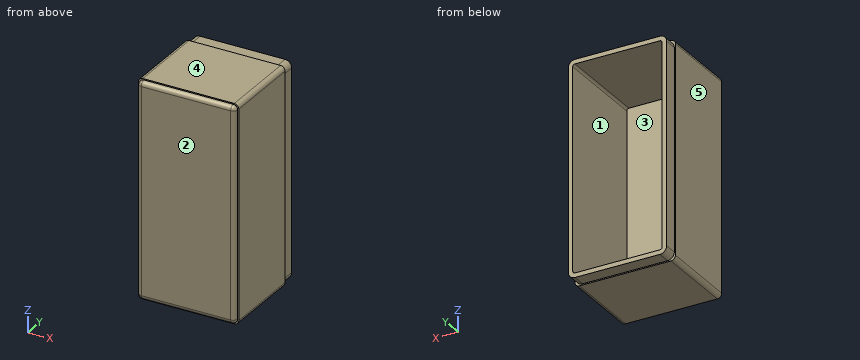
from build123d import *

# Parameters (mm, degrees)
SKETCH1_W           = 45
SKETCH1_H           = 97
BOSS_EXTRUDE1_DEPTH = 19
SKETCH2_W           = 44
SKETCH2_H           = 96
BOSS_EXTRUDE2_DEPTH = 6
SKETCH3_W           = 45
SKETCH3_H           = 97
SKETCH3_W_2         = 44
SKETCH3_H_2         = 96
CUT_EXTRUDE1_DEPTH  = 2
FILLET1_R           = 2
FILLET4_R           = 3
FILLET5_R           = 2
SHELL2_START        = -17
SHELL2_DEPTH        = 42
SHELL2_2_OUTLINE_W  = 41
SHELL2_2_OUTLINE_H  = 93
SHELL2_2_DEPTH      = 34
BOSS_EXTRUDE3_START = 34
SKETCH4_W           = 41
SKETCH4_H           = 93
BOSS_EXTRUDE3_DEPTH = 34


# Read off the part's stored shape, not the designer's step: Shell2
with BuildPart() as part:
    # Sketch1 → Boss-Extrude1 (new, symmetric)
    with BuildSketch(Plane(origin=(0, 0, 0), x_dir=(1, 0, 0), z_dir=(0, 1, 0))):
        Rectangle(SKETCH1_W, SKETCH1_H)
    extrude(amount=BOSS_EXTRUDE1_DEPTH, both=True)

    # Sketch2 → Boss-Extrude2 (add)
    with BuildSketch(Plane(origin=(0, 19, 0), x_dir=(1, 0, 0), z_dir=(0, 1, 0))):
        Rectangle(SKETCH2_W, SKETCH2_H)
    extrude(amount=BOSS_EXTRUDE2_DEPTH)

    # Sketch3 → Cut-Extrude1 (cut)
    with BuildSketch(Plane.XZ.offset(19)):
        Rectangle(SKETCH3_W, SKETCH3_H)
        Rectangle(SKETCH3_W_2, SKETCH3_H_2, mode=Mode.SUBTRACT)
    extrude(amount=-CUT_EXTRUDE1_DEPTH, mode=Mode.SUBTRACT)

    # Fillet1
    fillet1_edges = [part.edges().sort_by_distance(p)[0] for p in [
        (22, -19, 0),
        (22, -18, -48),
        (0, -19, -48),
        (-22, -18, -48),
        (-22, -19, 0),
        (-22, -18, 48),
        (0, -19, 48),
        (22, -18, 48),
    ]]
    fillet(fillet1_edges, radius=FILLET1_R - 0.0001)  # a hair under: the kernel refuses the full size

    # Fillet4
    fillet4_edges = [part.edges().sort_by_distance(p)[0] for p in [
        (22, 22, 48),
        (22, 22, -48),
        (-22, 22, -48),
        (-22, 22, 48),
    ]]
    fillet(fillet4_edges, radius=FILLET4_R)

    # Fillet5
    fillet5_edges = [part.edges().sort_by_distance(p)[0] for p in [
        (22.5, 1, 48.5),
        (-22.5, 1, 48.5),
        (-22.5, 1, -48.5),
        (22.5, 1, -48.5),
    ]]
    fillet(fillet5_edges, radius=FILLET5_R)

    # Shell2 outline → Shell2 (cut)
    with BuildSketch(Plane(origin=(0, 0, 0), x_dir=(1, 0, 0), z_dir=(0, 1, 0)).offset(SHELL2_START)):
        with BuildLine():
            Line((20, -45), (20, 45))
            ThreePointArc((20, 45), (19.707106781, 45.707106781), (19, 46))
            Line((19, 46), (-19, 46))
            ThreePointArc((-19, 46), (-19.707106781, 45.707106781), (-20, 45))
            Line((-20, 45), (-20, -45))
            ThreePointArc((-20, -45), (-19.707106781, -45.707106781), (-19, -46))
            Line((-19, -46), (19, -46))
            ThreePointArc((19, -46), (19.707106781, -45.707106781), (20, -45))
        make_face()
    extrude(amount=SHELL2_DEPTH, mode=Mode.SUBTRACT)

    # Shell2 2 outline → Shell2 2 (cut)
    with BuildSketch(Plane(origin=(0, 0, 0), x_dir=(1, 0, 0), z_dir=(0, 1, 0)).offset(SHELL2_START)):
        Rectangle(SHELL2_2_OUTLINE_W, SHELL2_2_OUTLINE_H)
        with BuildLine():
            ThreePointArc((19, 46), (19.707106781, 45.707106781), (20, 45))
            Line((20, 45), (20, -45))
            ThreePointArc((20, -45), (19.707106781, -45.707106781), (19, -46))
            Line((19, -46), (-19, -46))
            ThreePointArc((-19, -46), (-19.707106781, -45.707106781), (-20, -45))
            Line((-20, -45), (-20, 45))
            ThreePointArc((-20, 45), (-19.707106781, 45.707106781), (-19, 46))
            Line((-19, 46), (19, 46))
        make_face(mode=Mode.SUBTRACT)
    extrude(amount=SHELL2_2_DEPTH, mode=Mode.SUBTRACT)

    # Sketch4 → Boss-Extrude3 (add)
    with BuildSketch(Plane.XZ.offset(-17).offset(BOSS_EXTRUDE3_START)):
        Rectangle(SKETCH4_W, SKETCH4_H)
        with BuildLine():
            Line((19, -46), (-19, -46))
            ThreePointArc((-19, -46), (-19.707106781, -45.707106781), (-20, -45))
            Line((-20, -45), (-20, 45))
            ThreePointArc((-20, 45), (-19.707106781, 45.707106781), (-19, 46))
            Line((-19, 46), (19, 46))
            ThreePointArc((19, 46), (19.707106781, 45.707106781), (20, 45))
            Line((20, 45), (20, -45))
            ThreePointArc((20, -45), (19.707106781, -45.707106781), (19, -46))
        make_face(mode=Mode.SUBTRACT)
    extrude(amount=-BOSS_EXTRUDE3_DEPTH)


solid = part.part
Source: CAD feature listing. Evaluate the final solid. Frame: model axes, mm. Face numbers are marked on the shaded views. A direction names the side the tool comes from. Coordinates: 2 decimals unless noted, no trailing zeros. Order: outer loops, then holes, each group sorted by start corner. A loop starts at its lowest first (then second) coordinate and runs counter-clockwise, first axis right, second up.
Item 1: Pull-direction query (X, two-part tool) for the marked faces 3, 4 and 5; classes: pulls with the +X half, pulls with the -X half, needs draft (parallel to the pull), parting line crosses it, or undercut.
Output values:
face 3: undercut
face 4: needs draft
face 5: pulls with the -X half
Item 2: Material intervals for line 1 (Z direction, x = 17.5, y = -1.5); line 2 (X direction, y = 10, z = 20.5); line 3 (X direction, y = 21, z = 7.5), sorted ascending.
Output values:
line 1: z = -48.5 to -46, 46 to 48.5
line 2: x = -22.5 to -20, 20 to 22.5
line 3: x = -22 to -20, 20 to 22
Item 3: Cut plane A-A (y = 22.5). Return loops of the section in (x, z), plus the area to 3 significant figures.
Output values:
outline: (-22, -45) arc R3 ccw to (-19, -48) - (19, -48) arc R3 ccw to (22, -45) - (22, 45) arc R3 ccw to (19, 48) - (-19, 48) arc R3 ccw to (-22, 45) - close; hole (-20, -45) arc R1 ccw to (-19, -46) - (19, -46) arc R1 ccw to (20, -45) - (20, 45) arc R1 ccw to (19, 46) - (-19, 46) arc R1 ccw to (-20, 45) - close
area: 537 mm2
Item 4: Cut plane D-D (y = 14). Return loops of the section in (x, z).
Output values:
outline: (-22.5, -46.5) arc R2 ccw to (-20.5, -48.5) - (20.5, -48.5) arc R2 ccw to (22.5, -46.5) - (22.5, 46.5) arc R2 ccw to (20.5, 48.5) - (-20.5, 48.5) arc R2 ccw to (-22.5, 46.5) - close; hole (-20, -45) arc R1 ccw to (-19, -46) - (19, -46) arc R1 ccw to (20, -45) - (20, 45) arc R1 ccw to (19, 46) - (-19, 46) arc R1 ccw to (-20, 45) - close
Item 5: First-contact query: P1, Ø1.8, axis at y = 21.5, z = 21.5, coming from the -X side. Flat tip, straight axial feed; report the tip coordinate or a pass-through.
Output values:
P1: stops at x = -22
Item 6: Set-up query: the marked faces 1 and 2. Return all of +Z, -Z, +X, -X, +Y, -Y with unobstructed straight access to the full face (end or side cutting, diameter ignored); none if empty.
Output values:
face 1: +Y
face 2: +Z, -Z, +X, -X, -Y
